```python
from build123d import *

# Parameters (mm, degrees)
SKETCH1_W           = 100
SKETCH1_H           = 100
BOSS_EXTRUDE1_DEPTH = 6
SKETCH2_R           = 2.9
CUT_EXTRUDE1_DEPTH  = 3.8
SKETCH3_R           = 1.7
CUT_EXTRUDE2_DEPTH  = 6
SKETCH4_R           = 2.3
CUT_EXTRUDE3_DEPTH  = 2.5
SKETCH5_R           = 1.4
CUT_EXTRUDE4_DEPTH  = 6
SKETCH6_W           = 100
SKETCH6_H           = 100
CUT_EXTRUDE5_DEPTH  = 10
CUT_EXTRUDE6_REACH  = 8


with BuildPart() as part:
    # Sketch1 → Boss-Extrude1 (new body)
    with BuildSketch(Plane.XY):
        with Locations((0, -30)):
            Rectangle(SKETCH1_W, SKETCH1_H)
    extrude(amount=BOSS_EXTRUDE1_DEPTH)

    # Sketch2 → Cut-Extrude1 (cut)
    with BuildSketch(Plane.XY):
        with Locations((21.1, -8)):
            Circle(SKETCH2_R)
        with Locations((-21.1, 8)):
            Circle(SKETCH2_R)
        with Locations((-21.1, -8)):
            Circle(SKETCH2_R)
        with Locations((21.1, 8)):
            Circle(SKETCH2_R)
    extrude(amount=CUT_EXTRUDE1_DEPTH, mode=Mode.SUBTRACT)

    # Sketch3 → Cut-Extrude2 (cut)
    with BuildSketch(Plane(origin=(0, 0, 0), x_dir=(-1, 0, 0), z_dir=(0, 0, -1))):
        with Locations((-21.1, 8)):
            Circle(SKETCH3_R)
        with Locations((21.1, 8)):
            Circle(SKETCH3_R)
        with Locations((21.1, -8)):
            Circle(SKETCH3_R)
        with Locations((-21.1, -8)):
            Circle(SKETCH3_R)
    extrude(amount=-CUT_EXTRUDE2_DEPTH, mode=Mode.SUBTRACT)

    # Sketch4 → Cut-Extrude3 (cut)
    with BuildSketch(Plane(origin=(0, 0, 0), x_dir=(-1, 0, 0), z_dir=(0, 0, -1))):
        with Locations((-38, -59)):
            Circle(SKETCH4_R)
        with Locations((-38, -51)):
            Circle(SKETCH4_R)
        with Locations((-22, -51)):
            Circle(SKETCH4_R)
        with Locations((-22, -59)):
            Circle(SKETCH4_R)
        with Locations((37.999999976, -59)):
            Circle(SKETCH4_R)
        with Locations((22, -51)):
            Circle(SKETCH4_R)
        with Locations((22, -59)):
            Circle(SKETCH4_R)
        with Locations((37.999999976, -51)):
            Circle(SKETCH4_R)
    extrude(amount=-CUT_EXTRUDE3_DEPTH, mode=Mode.SUBTRACT)

    # Sketch5 → Cut-Extrude4 (cut)
    with BuildSketch(Plane(origin=(0, 0, 0), x_dir=(-1, 0, 0), z_dir=(0, 0, -1))):
        with Locations((-38.000000024, -59)):
            Circle(SKETCH5_R)
        with Locations((-38.000000024, -51)):
            Circle(SKETCH5_R)
        with Locations((-22, -51)):
            Circle(SKETCH5_R)
        with Locations((-22, -59)):
            Circle(SKETCH5_R)
        with Locations((37.999999976, -59)):
            Circle(SKETCH5_R)
        with Locations((22, -51)):
            Circle(SKETCH5_R)
        with Locations((22, -59)):
            Circle(SKETCH5_R)
        with Locations((37.999999976, -51)):
            Circle(SKETCH5_R)
    extrude(amount=-CUT_EXTRUDE4_DEPTH, mode=Mode.SUBTRACT)

    # Sketch6 → Cut-Extrude5 (cut)
    with BuildSketch(Plane.XY.offset(6)):
        with Locations((0, -30)):
            Rectangle(SKETCH6_W, SKETCH6_H)
        with BuildLine():
            Line((-31.1, -14), (-31.1, 14))
            ThreePointArc((-31.1, 14), (-29.928427125, 16.828427125), (-27.1, 18))
            Line((-27.1, 18), (27.1, 18))
            ThreePointArc((27.1, 18), (29.928427125, 16.828427125), (31.1, 14))
            Line((31.1, 14), (31.1, -14))
            ThreePointArc((31.1, -14), (29.928427125, -16.828427125), (27.1, -18))
            Line((27.1, -18), (14, -18))
            ThreePointArc((14, -18), (11.171572875, -19.171572875), (10, -22))
            Line((10, -22), (10, -37))
            ThreePointArc((10, -37), (11.171572875, -39.828427125), (14, -41))
            Line((14, -41), (44.000000024, -41))
            ThreePointArc((44.000000024, -41), (46.828427149, -42.171572875), (48.000000024, -45))
            Line((48.000000024, -45), (48.000000024, -65))
            ThreePointArc((48.000000024, -65), (46.828427149, -67.828427125), (44.000000024, -69))
            Line((44.000000024, -69), (-43.999999976, -69))
            ThreePointArc((-43.999999976, -69), (-46.8284271, -67.828427125), (-47.999999976, -65))
            Line((-47.999999976, -65), (-47.999999976, -45))
            ThreePointArc((-47.999999976, -45), (-46.8284271, -42.171572875), (-43.999999976, -41))
            Line((-43.999999976, -41), (-14, -41))
            ThreePointArc((-14, -41), (-11.171572875, -39.828427125), (-10, -37))
            Line((-10, -37), (-10, -22))
            ThreePointArc((-10, -22), (-11.171572875, -19.171572875), (-14, -18))
            Line((-14, -18), (-27.1, -18))
            ThreePointArc((-27.1, -18), (-29.928427125, -16.828427125), (-31.1, -14))
        make_face(mode=Mode.SUBTRACT)
    extrude(amount=-CUT_EXTRUDE5_DEPTH, mode=Mode.SUBTRACT)

    # Sketch7 → Cut-Extrude6 (cut, up to next)
    with BuildSketch(Plane.XY, mode=Mode.PRIVATE) as cut_extrude6_sk1:
        with BuildLine():
            Line((-11.1, 18), (-11.1, -3))
            ThreePointArc((-11.1, -3), (-10.221320344, -5.121320344), (-8.1, -6))
            Line((-8.1, -6), (8.1, -6))
            ThreePointArc((8.1, -6), (10.221320344, -5.121320344), (11.1, -3))
            Line((11.1, -3), (11.1, 18))
            Line((11.1, 18), (-11.1, 18))
        make_face()
    cut_extrude6_tool1 = extrude(cut_extrude6_sk1.sketch, amount=CUT_EXTRUDE6_REACH, mode=Mode.PRIVATE) & part.part
    add(cut_extrude6_tool1.solids().sort_by_distance((0, 6.082742, 0))[0], mode=Mode.SUBTRACT)


solid = part.part
```
For this review, take the finished solid that the model builds, in its own axes (mm). A direction names the side the tool comes from. Give positions to 0.01 mm unless a question says otherwise; leave off trailing zeros. Write each loop counter-clockwise with the first axis right and the second up, starting at its lowest first coordinate (ties: lowest second). Pieces come first, ordered by that corner, then holes. Notation, with made-up numbers: M 41.5,60 L 64.5,60 A23 ccw 64.5,93 Z; hole C 82.25,80.25 d11. An arc over 180 degrees is marked long. One line per item, written item: value.
1) Take a section at D-D, the plane x = -29. Write out the cut boundary in (y, z).
Results are:
outline: M -69,0 L -41,0 L -41,6 L -69,6 Z; M -17.52,0 L 17.52,0 L 17.52,6 L -17.52,6 Z
2) For P1, Ø3, axis at x = 0.5, z = 4, coming from the +Y side; P2, Ø1.8, axis at y = 11.5, z = 3, coming from the -X side; P3, Ø3.5, axis at x = 22.5, y = -51, coming from the -Z side; P4, Ø12, axis at x = -37, y = -17, coming from the +Z side, all flat-tipped, find the tip position at first contact; note any pin that passes through.
Results are:
P1: stops at y = -6
P2: stops at x = -31.1
P3: stops at z = 2.5
P4: passes through
3) For faces 5 (the flat face through (-20, -18, 3)), 6 (the cylindrical face through (11.203, -19.141, 3.042)), 7 (the flat face through (-11.1, 8, 3)), 8 (the flat face through (-38, -53, 2.5)), list the 3-axis set-ups (+Z, -Z, +X, -X, +Y, -Y) from which the entire face can be reached by the end or side of a thin tool; tool diameter is ignored.
Results are:
face 5: +Z, -Z, -X
face 6: +Z, -Z, +X
face 7: +Z, -Z, +Y
face 8: -Z
4) The part is to be moulded in two halves that separate along X. For faces 1 (the flat face through (19, 18, 3)), 2 (the cylindrical face through (38.499, -61.245, 1.232)), 3 (the flat face through (48, -55, 3)), 4 (the cylindrical face through (-18.334, -7.129, 1.873)), say which applies: +X half, -X half, draft (parallel to the pull), parting line (faces both ways), or undercut.
Results are:
face 1: draft
face 2: undercut
face 3: +X half
face 4: undercut
5) For line 1 (Y direction, x = -38, z = 4.3); line 2 (X direction, y = -60.5, z = 1.35); line 3 (Y direction, x = 15.5, z = 4.45), list the stretches that pass through material, from the lowest coordinate up. Write a range as from..to.
Results are:
line 1: y = -69..-60.4, -57.6..-52.4, -49.6..-41
line 2: x = -48..-39.74, -36.26..-23.74, -20.26..20.26, 23.74..36.26, 39.74..48
line 3: y = -69..-41, -18..18
6) Take a section at B-B, the plane y = -59. Count the separate pieces of the cut face and the enclosed holes in it, then the cut area to 3 significant figures.
Results are:
separate pieces: 5
enclosed holes: 0
area: 491 mm²
7) Take a section at C-C, the plane y = -12. Write out the cut boundary in (x, z), then the cut area to 3 significant figures.
Results are:
outline: M -31.1,0 L 31.1,0 L 31.1,6 L -31.1,6 Z
area: 373 mm²
8) Take a section at A-A, the plane x = 17. Write out the cut boundary in (y, z).
Results are:
outline: M -69,0 L -41,0 L -41,6 L -69,6 Z; M -18,0 L 18,0 L 18,6 L -18,6 Z
